Verification items for the finished model (mm, model axes). A direction names the side the tool comes from. Coordinates: 2 decimals unless noted, no trailing zeros. Order: outer loops, then holes, each group sorted by start corner. A loop starts at its lowest first (then second) coordinate and runs counter-clockwise, first axis right, second up. Notation, with made-up numbers: (89.25, -24) -> (130.25, -24) arc R17 cw to (130.25, -9) -> close; hole circle Ø4 at (66.5, 11). An arc over 180 degrees is marked (long way). Write each question's results on one line, items separated by ' | '. Start each with the question number.
(1) Go/stop test with flat-tipped pins: pin 1 (4 mm diameter, centred on y = 33, z = -2.5, fed in from +X); pin 2 (2.5 mm diameter, centred on x = -0.5, z = 0.5, fed in from +Y); pin 3 (2 mm diameter, centred on y = 19.5, z = 3.5, fed in from +X). Record where each tip stops, or that it passes through.
(2) Draft check along X on faces 4 (the cylindrical face through (-1.66, 4.68, -0.37)), 5 (the cylindrical face through (-1.66, 44.27, -0.37)), 6 (the flat face through (1.35, 49.2, 1.35)). Enter one of: +X half, -X half, draft (parallel to the pull), parting line (faces both ways), or undercut.
(3) Cross-section at B-B on x = 0. Enter the section's corners in (y, z).
(4) Cross-section at D-D on y = 37. Enter the section's corners in (x, z), and give its area (3 significant figures).
(5) Cross-section at A-A on z = 0. Enter the section's corners in (x, y).
(6) Thickness scan on probe 1 along X at (y, z) = (45.5, 0); probe 2 along Z at (x, y) = (0.75, 47); probe 3 along Y at (x, z) = (2.25, 1.25). Record the ranges inside material, lowest first. Write a range as [from, to].
(7) Set-up check for faces 1 (the flat face through (0, 39.2, 0)), 2 (the flat face through (-2.5, 10, -0.1)), 3 (the flat face through (0, 0, 0)): record each of +Z, -Z, +X, -X, +Y, -Y from which the full face is reachable in a straight line by a thin tool's end or side.
(8) Cross-section at C-C on y = 43. Enter the section's corners in (x, z).
```python
from build123d import *


with BuildPart() as part:
    # Esboço1 → Revolução1 (revolve)
    with BuildSketch(Plane(origin=(0, 0, 0), x_dir=(-1, 0, 0), z_dir=(0, 0, -1)), mode=Mode.PRIVATE) as revolu_o1_sk:
        with BuildLine():
            Line((-1.7, 0), (0, 0))
            Line((0, 0), (0, 39.2))
            Line((0, 39.2), (-1.7, 39.2))
            Line((-1.7, 39.2), (-1.7, 49.2))
            Line((-1.7, 49.2), (-5.7, 49.2))
            Line((-5.7, 49.2), (-6, 48.9))
            Line((-6, 48.9), (-6, 10.3))
            Line((-6, 10.3), (-5.7, 10))
            Line((-5.7, 10), (-2.2, 10))
            ThreePointArc((-2.2, 10), (-1.846446609, 9.853553391), (-1.7, 9.5))
            Line((-1.7, 9.5), (-1.7, 0))
        make_face()
    revolve(revolu_o1_sk.sketch.rotate(Axis((0, 0, 0), (0, 1, 0)), 270), axis=Axis((0, 0, 0), (0, 1, 0)))


solid = part.part
```
Results are:
1) pin 1: stops at x = 5.98 | pin 2: stops at y = 49.2 | pin 3: stops at x = 5.45
2) face 4: parting line | face 5: undercut | face 6: draft
3) outline: (0, -1.7) -> (9.5, -1.7) arc R0.5 cw to (10, -2.2) -> (10, -5.7) -> (10.3, -6) -> (48.9, -6) -> (49.2, -5.7) -> (49.2, -1.7) -> (39.2, -1.7) -> (39.2, 1.7) -> (49.2, 1.7) -> (49.2, 5.7) -> (48.9, 6) -> (10.3, 6) -> (10, 5.7) -> (10, 2.2) arc R0.5 cw to (9.5, 1.7) -> (0, 1.7) -> close
4) outline: circle Ø12 at (0, 0) | area: 113 mm2
5) outline: (-6, 10.3) -> (-5.7, 10) -> (-2.2, 10) arc R0.5 cw to (-1.7, 9.5) -> (-1.7, 0) -> (1.7, 0) -> (1.7, 9.5) arc R0.5 cw to (2.2, 10) -> (5.7, 10) -> (6, 10.3) -> (6, 48.9) -> (5.7, 49.2) -> (1.7, 49.2) -> (1.7, 39.2) -> (-1.7, 39.2) -> (-1.7, 49.2) -> (-5.7, 49.2) -> (-6, 48.9) -> close
6) probe 1: x = [-6, -1.7], [1.7, 6] | probe 2: z = [-5.95, -1.53], [1.53, 5.95] | probe 3: y = [10, 49.2]
7) face 1: +Y | face 2: -Y | face 3: +Z, -Z, +X, -X, -Y
8) outline: circle Ø12 at (0, 0); hole circle Ø3.4 at (0, 0)
